from build123d import *

# Parameters (mm, degrees)
ESBO_O1_W                = 215.5
ESBO_O1_H                = 160
RESSALTO_EXTRUS_O1_DEPTH = 90
ESBO_O2_W                = 93
ESBO_O2_H                = 60
RESSALTO_EXTRUS_O2_DEPTH = 80
CORTE_EXTRUS_O1_REACH    = 241.777
ESBO_O4_R                = 2.5
ESBO_O4_R_2              = 2.72809557
CORTE_EXTRUS_O2_DEPTH    = 5
ESBO_O5_W                = 215.5
ESBO_O5_H                = 160
ESBO_O5_W_2              = 195.5
ESBO_O5_H_2              = 140
RESSALTO_EXTRUS_O3_DEPTH = 3
ESBO_O6_R                = 4
CORTE_EXTRUS_O3_DEPTH    = 10


with BuildPart() as part:
    # Esboço1 → Ressalto-extrusão1 (new body)
    with BuildSketch(Plane(origin=(0, 0, 0), x_dir=(1, 0, 0), z_dir=(0, 1, 0))):
        Rectangle(ESBO_O1_W, ESBO_O1_H)
    extrude(amount=RESSALTO_EXTRUS_O1_DEPTH)

    # Esboço2 → Ressalto-extrusão2 (add)
    with BuildSketch(Plane.XY.offset(80)):
        with Locations((0, 30)):
            Rectangle(ESBO_O2_W, ESBO_O2_H)
    extrude(amount=RESSALTO_EXTRUS_O2_DEPTH)

    # Esboço3 → Corte-extrusão1 (cut, up to next)
    with BuildSketch(Plane.ZY.offset(46.5), mode=Mode.PRIVATE) as corte_extrus_o1_sk1:
        Polygon((160, 60), (160, 40), (80, 60), align=None)
    corte_extrus_o1_tool1 = extrude(corte_extrus_o1_sk1.sketch, amount=-CORTE_EXTRUS_O1_REACH, mode=Mode.PRIVATE) & part.part
    add(corte_extrus_o1_tool1.solids().sort_by_distance((-46.5, 53.333333, 133.333333))[0], mode=Mode.SUBTRACT)

    # Esboço4 → Corte-extrusão2 (cut)
    with BuildSketch(Plane(origin=(0, 75.294117647, 18.823529412), x_dir=(1, 0, 0), z_dir=(0, 0.9701425001453319, 0.24253562503633308))):
        with Locations(Location((0, -115.409748765, 0), (0, 0, 270))):
            Circle(ESBO_O4_R)
        with Locations(Location((-15, -104.290318766, 0), (0, 0, 270))):
            Circle(ESBO_O4_R)
        with Locations(Location((0, -93.170888766, 0), (0, 0, 270))):
            Circle(ESBO_O4_R)
        with Locations(Location((0, -104.290318766, 0), (0, 0, 270))):
            Circle(ESBO_O4_R)
        with Locations(Location((15, -104.290318766, 0), (0, 0, 270))):
            Circle(ESBO_O4_R_2)
    extrude(amount=-CORTE_EXTRUS_O2_DEPTH, mode=Mode.SUBTRACT)

    # Esboço5 → Ressalto-extrusão3 (add)
    with BuildSketch(Plane(origin=(0, 90, 0), x_dir=(1, 0, 0), z_dir=(0, 1, 0))):
        Rectangle(ESBO_O5_W, ESBO_O5_H)
        Rectangle(ESBO_O5_W_2, ESBO_O5_H_2, mode=Mode.SUBTRACT)
    extrude(amount=RESSALTO_EXTRUS_O3_DEPTH)

    # Esboço6 → Corte-extrusão3 (cut)
    with BuildSketch(Plane(origin=(0, 90, 0), x_dir=(1, 0, 0), z_dir=(0, 1, 0))):
        with Locations(Location((-81, 54, 0), (0, 0, 270))):
            Circle(ESBO_O6_R)
        with Locations(Location((-54, 54, 0), (0, 0, 270))):
            Circle(ESBO_O6_R)
        with Locations(Location((-27, 54, 0), (0, 0, 270))):
            Circle(ESBO_O6_R)
        with Locations(Location((0, 54, 0), (0, 0, 270))):
            Circle(ESBO_O6_R)
        with Locations(Location((27, 54, 0), (0, 0, 270))):
            Circle(ESBO_O6_R)
        with Locations(Location((54, 54, 0), (0, 0, 270))):
            Circle(ESBO_O6_R)
        with Locations(Location((81, 54, 0), (0, 0, 270))):
            Circle(ESBO_O6_R)
        with Locations(Location((81, 27, 0), (0, 0, 270))):
            Circle(ESBO_O6_R)
        with Locations(Location((54, 27, 0), (0, 0, 270))):
            Circle(ESBO_O6_R)
        with Locations(Location((27, 27, 0), (0, 0, 270))):
            Circle(ESBO_O6_R)
        with Locations(Location((0, 27, 0), (0, 0, 270))):
            Circle(ESBO_O6_R)
        with Locations(Location((-27, 27, 0), (0, 0, 270))):
            Circle(ESBO_O6_R)
        with Locations(Location((-54, 27, 0), (0, 0, 270))):
            Circle(ESBO_O6_R)
        with Locations(Location((-81, 27, 0), (0, 0, 270))):
            Circle(ESBO_O6_R)
        with Locations(Location((-81, 0, 0), (0, 0, 270))):
            Circle(ESBO_O6_R)
        with Locations(Location((-54, 0, 0), (0, 0, 270))):
            Circle(ESBO_O6_R)
        with Locations(Location((-27, 0, 0), (0, 0, 270))):
            Circle(ESBO_O6_R)
        with Locations(Location((0, 0, 0), (0, 0, 270))):
            Circle(ESBO_O6_R)
        with Locations(Location((27, 0, 0), (0, 0, 270))):
            Circle(ESBO_O6_R)
        with Locations(Location((54, 0, 0), (0, 0, 270))):
            Circle(ESBO_O6_R)
        with Locations(Location((81, 0, 0), (0, 0, 270))):
            Circle(ESBO_O6_R)
        with Locations(Location((81, -27, 0), (0, 0, 270))):
            Circle(ESBO_O6_R)
        with Locations(Location((54, -27, 0), (0, 0, 270))):
            Circle(ESBO_O6_R)
        with Locations(Location((27, -27, 0), (0, 0, 270))):
            Circle(ESBO_O6_R)
        with Locations(Location((0, -27, 0), (0, 0, 270))):
            Circle(ESBO_O6_R)
        with Locations(Location((-27, -27, 0), (0, 0, 270))):
            Circle(ESBO_O6_R)
        with Locations(Location((-54, -27, 0), (0, 0, 270))):
            Circle(ESBO_O6_R)
        with Locations(Location((-81, -27, 0), (0, 0, 270))):
            Circle(ESBO_O6_R)
        with Locations(Location((-81, -54, 0), (0, 0, 270))):
            Circle(ESBO_O6_R)
        with Locations(Location((-54, -54, 0), (0, 0, 270))):
            Circle(ESBO_O6_R)
        with Locations(Location((-27, -54, 0), (0, 0, 270))):
            Circle(ESBO_O6_R)
        with Locations(Location((0, -54, 0), (0, 0, 270))):
            Circle(ESBO_O6_R)
        with Locations(Location((27, -54, 0), (0, 0, 270))):
            Circle(ESBO_O6_R)
        with Locations(Location((54, -54, 0), (0, 0, 270))):
            Circle(ESBO_O6_R)
        with Locations(Location((81, -54, 0), (0, 0, 270))):
            Circle(ESBO_O6_R)
    extrude(amount=-CORTE_EXTRUS_O3_DEPTH, mode=Mode.SUBTRACT)


solid = part.part
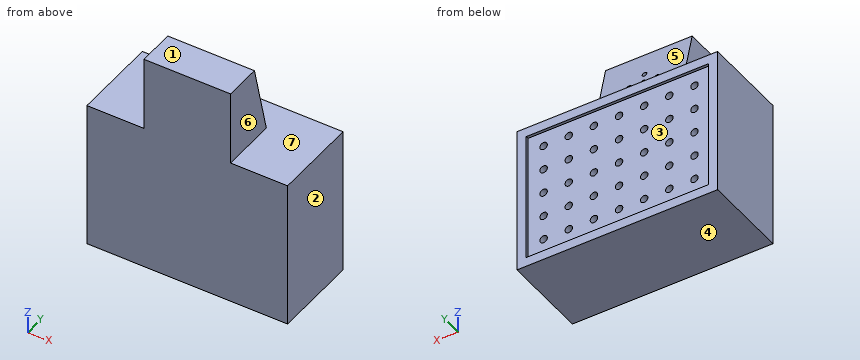
For this review, take the finished solid that the model builds, in its own axes (mm). Face numbers are marked on the shaded views. A direction names the side the tool comes from. Round coordinates to 2 decimals unless told otherwise and drop trailing zeros. Order: outer loops, then holes, each group sorted by start corner. A loop starts at its lowest first (then second) coordinate and runs counter-clockwise, first axis right, second up. Notation, with made-up numbers: (23, 52.25) -> (52, 52.25) arc R20 cw to (52, 69.25) -> close; hole circle Ø8 at (87.5, 36). An arc over 180 degrees is marked (long way). Write item = value, one per line. Start each with the question number.
1) Insertion check: pin 1 (4 mm diameter, centred on x = -84, y = 69, fed in from +Z); pin 2 (9 mm diameter, centred on x = -28, z = 52.5, fed in from +Y); pin 3 (4 mm diameter, centred on x = 28, z = -27, fed in from +Y). Each pin has a flat end and moves straight along its axis. Give the tip position at first contact, or say it passes through.
2) To check wall thickness, follow line 1 (Y direction, x = 95, z = -56.5); line 2 (Z direction, x = 70, y = 4.5); line 3 (X direction, y = 23.5, z = 143). State the ranges of each line that lie inside material, in increasing order. Write a range as from..to.
3) Tool access review of the marked faces 5, 6 and 7: name each direction out of +Z, -Z, +X, -X, +Y, -Y from which nothing blocks a thin tool from reaching the whole face with its end or side.
4) The part is to be moulded in two halves that separate along Z. For the marked faces 1, 2, 3 and 4, say which applies: +Z half, -Z half, draft (parallel to the pull), parting line (faces both ways), or undercut.
5) Take a section at A-A on x = -42.5. State the section outline as (y, z) points.
6) Take a section at C-C on z = -61.5. State the section outline as (x, y) points, plus the area to 3 significant figures.
7) Take a section at B-B on y = 9. State the section outline as (x, z) points.
8) Take a section at D-D on x = 54. State the section outline as (y, z) points, plus the area to 3 significant figures.
Verdict:
q1.pin_1 = 80
q1.pin_2 = 90
q1.pin_3 = 80
q2.line_1 = 0..90
q2.line_2 = -80..80
q2.line_3 = -46.5..46.5
q3.face_5 = +Z, +X, -X, +Y
q3.face_6 = +Z, +X, +Y, -Y
q3.face_7 = +Z, +Y
q4.face_1 = +Z half
q4.face_2 = draft
q4.face_3 = undercut
q4.face_4 = -Z half
q5.outline = (0, -80) -> (93, -80) -> (93, -70) -> (90, -70) -> (90, 70) -> (93, 70) -> (93, 80) -> (60, 80) -> (40, 160) -> (0, 160) -> close
q6.outline = (-107.75, 0) -> (107.75, 0) -> (107.75, 93) -> (97.75, 93) -> (97.75, 90) -> (-97.75, 90) -> (-97.75, 93) -> (-107.75, 93) -> close
q6.area = 19,500 mm2
q7.outline = (-107.75, -80) -> (107.75, -80) -> (107.75, 80) -> (46.5, 80) -> (46.5, 160) -> (-46.5, 160) -> (-46.5, 80) -> (-107.75, 80) -> close
q8.outline = (0, -80) -> (93, -80) -> (93, -70) -> (90, -70) -> (90, -58) -> (80, -58) -> (80, -50) -> (90, -50) -> (90, -31) -> (80, -31) -> (80, -23) -> (90, -23) -> (90, -4) -> (80, -4) -> (80, 4) -> (90, 4) -> (90, 23) -> (80, 23) -> (80, 31) -> (90, 31) -> (90, 50) -> (80, 50) -> (80, 58) -> (90, 58) -> (90, 70) -> (93, 70) -> (93, 80) -> (0, 80) -> close
q8.area = 14,100 mm2
